The listing builds one solid part. Answer for the finished solid, in the listing's coordinates (mm). A direction names the side the tool comes from. Give positions to 0.01 mm unless a question says otherwise; leave off trailing zeros. Write each loop counter-clockwise with the first axis right and the second up, starting at its lowest first coordinate (ties: lowest second). Pieces come first, ordered by that corner, then holes. Notation, with made-up numbers: M -38.5,26.25 L -13.5,26.25 A26 ccw -13.5,43.25 Z; hole C 73.25,26.5 d9. An arc over 180 degrees is marked long. Answer as a JSON object with one key per item and string values.
```python
from build123d import *

# Parameters (mm, degrees)
BOSS_EXTRUDE1_DEPTH     = 50
BOSS_EXTRUDE1_2_DEPTH   = 50
BOSS_EXTRUDE2_DEPTH     = 10
CHAMFER1_SIZE           = 15
CHAMFER1_SIZE_2         = 20
SKETCH4_W               = 160
SKETCH4_H               = 200
BOSS_EXTRUDE3_DEPTH     = 5
FILLET1_R               = 10
SKETCH5_R               = 7.5
CUT_EXTRUDE1_DEPTH      = 5
CUT_EXTRUDE5_DEPTH      = 140.373598648
CUT_EXTRUDE5_DEPTH_BACK = 140.373598648
FILLET4_R               = 5
SKETCH12_R              = 2
CUT_EXTRUDE6_DEPTH      = 10


with BuildPart() as part:
    # Sketch2 → Boss-Extrude1 (new body)
    with BuildSketch(Plane.XY):
        with BuildLine():
            Line((-50, 75), (-22.70223243, 0))
            Line((-22.70223243, 0), (-37.64392369, -17.092022104))
            ThreePointArc((-37.64392369, -17.092022104), (-49.971924127, -51.675350432), (-35.355339059, -85.355339059))
            Line((-35.355339059, -85.355339059), (-35.355339059, -100))
            Line((-35.355339059, -100), (-80, -100))
            Line((-80, -100), (-80, 100))
            Line((-80, 100), (-50, 100))
            Line((-50, 100), (-50, 75))
        make_face()
    extrude(amount=-BOSS_EXTRUDE1_DEPTH)



with BuildPart() as body_2:
    # Sketch2 → Boss-Extrude1 2 (new body)
    with BuildSketch(Plane.XY):
        with BuildLine():
            Line((50, 75), (22.70223243, 0))
            Line((22.70223243, 0), (37.64392369, -17.092022104))
            ThreePointArc((37.64392369, -17.092022104), (49.971924127, -51.675350432), (35.355339059, -85.355339059))
            Line((35.355339059, -85.355339059), (35.355339059, -100))
            Line((35.355339059, -100), (80, -100))
            Line((80, -100), (80, 100))
            Line((80, 100), (50, 100))
            Line((50, 100), (50, 75))
        make_face()
    extrude(amount=-BOSS_EXTRUDE1_2_DEPTH)


with BuildPart() as part_1:
    add(part.part)

    add(body_2.part)  # Boss-Extrude2 merges body 2
    # Sketch3 → Boss-Extrude2 (add)
    with BuildSketch(Plane.XY):
        Polygon((-29.981637115, 20), (29.981637115, 20), (22.70223243, 0), (-22.70223243, 0), align=None)
    extrude(amount=-BOSS_EXTRUDE2_DEPTH)

    # Chamfer1
    # the kernel refuses this chamfer: 20, 15 mm, written as the material it takes off along each edge
    with BuildSketch(Plane(origin=(-81.595588718, 20, -10), x_dir=(0, 0.041308380137954244, 0.9991464445867674), z_dir=(1, 0, 0))) as chamfer1_piece_1_section:
        Polygon((CHAMFER1_SIZE * 0.999146444587, CHAMFER1_SIZE * 0.041308380138), (-CHAMFER1_SIZE_2 * 0.041308380138, CHAMFER1_SIZE_2 * 0.999146444587), (0, 0), align=None)
    chamfer1_piece_1 = extrude(amount=163.191177435, mode=Mode.PRIVATE)
    chamfer1_piece_1 = split(chamfer1_piece_1, bisect_by=Plane(origin=(-24.447399798, 4.794807938, -4.975922198), z_dir=(0.9396926207859094, 0.3420201433256661, 0)), keep=Keep.TOP, mode=Mode.PRIVATE)
    chamfer1_piece_1 = split(chamfer1_piece_1, bisect_by=Plane(origin=(24.447399798, 4.794807938, -4.975922198), z_dir=(-0.939692620785907, 0.34202014332567265, 0)), keep=Keep.TOP, mode=Mode.PRIVATE)
    add(chamfer1_piece_1, mode=Mode.SUBTRACT)

    # Sketch4 → Boss-Extrude3 (add)
    with BuildSketch(Plane.XY):
        Rectangle(SKETCH4_W, SKETCH4_H)
    extrude(amount=BOSS_EXTRUDE3_DEPTH)

    # Fillet1
    fillet1_edges = [part_1.edges().sort_by_distance(p)[0] for p in [
        (-22.70223243, 0, -30),
        (-35.355339059, -85.355339059, -25),
        (35.355339059, -85.355339059, -25),
        (22.70223243, 0, -30),
        (0, 13.333333333, 0),
    ]]
    fillet(fillet1_edges, radius=FILLET1_R)

    # Sketch5 → Cut-Extrude1 (cut)
    with BuildSketch(Plane(origin=(0, 0, 0), x_dir=(-1, 0, 0), z_dir=(0, 0, -1))):
        with Locations((0, -50)):
            Circle(SKETCH5_R)
    extrude(amount=-CUT_EXTRUDE1_DEPTH, mode=Mode.SUBTRACT)

    # Sketch11 → Cut-Extrude5 (cut, two sides: drawn at the far end of the back side and taken through both)
    with BuildSketch(Plane(origin=(0, 0, -50), x_dir=(-1, 0, 0), z_dir=(0, 0, -1)).offset(-CUT_EXTRUDE5_DEPTH_BACK)):
        with BuildLine():
            Line((-58.784198233, -62.017405631), (-51.672968794, -96.802610845))
            ThreePointArc((-51.672968794, -96.802610845), (-51.161121522, -98.466118532), (-50.338653833, -100))
            Line((-50.338653833, -100), (-80, -100))
            Line((-80, -100), (-80, 100))
            Line((-80, 100), (-62.474937186, 100))
            ThreePointArc((-62.474937186, 100), (-66.199502533, 94.806221081), (-65.536970349, 88.4494312))
            Line((-65.536970349, 88.4494312), (-60, 73.236730193))
            Line((-60, 73.236730193), (-34.120235365, 2.132661237))
            Line((-34.120235365, 2.132661237), (-45.172708428, -10.510426525))
            ThreePointArc((-45.172708428, -10.510426525), (-58.008635864, -34.670350128), (-58.784198233, -62.017405631))
        make_face()
        with BuildLine():
            Line((34.120235365, 2.132661237), (45.172708428, -10.510426525))
            ThreePointArc((45.172708428, -10.510426525), (58.008635864, -34.670350128), (58.784198233, -62.017405631))
            Line((58.784198233, -62.017405631), (51.672968794, -96.802610845))
            ThreePointArc((51.672968794, -96.802610845), (51.161121522, -98.466118532), (50.338653833, -100))
            Line((50.338653833, -100), (80, -100))
            Line((80, -100), (80, 100))
            Line((80, 100), (62.474937186, 100))
            ThreePointArc((62.474937186, 100), (66.199502533, 94.806221081), (65.536970349, 88.4494312))
            Line((65.536970349, 88.4494312), (60, 73.236730193))
            Line((60, 73.236730193), (34.120235365, 2.132661237))
        make_face()
    extrude(amount=CUT_EXTRUDE5_DEPTH + CUT_EXTRUDE5_DEPTH_BACK, mode=Mode.SUBTRACT)

    # Fillet4
    fillet4_edges = [part_1.edges().sort_by_distance(p)[0] for p in [
        (-35.355339059, -100, -25),
        (-50, 100, -25),
        (62.474937186, 100, -22.5),
        (-62.474937186, 100, -22.5),
        (50, 100, -25),
        (35.355339059, -100, -25),
    ]]
    fillet(fillet4_edges, radius=FILLET4_R)

    # Sketch12 → Cut-Extrude6 (cut)
    with BuildSketch(Plane(origin=(0, 0, -50), x_dir=(-1, 0, 0), z_dir=(0, 0, -1))):
        with Locations((-57.5, 92.5)):
            Circle(SKETCH12_R)
        with Locations((57.5, 92.5)):
            Circle(SKETCH12_R)
        with Locations((-42.855339059, -95)):
            Circle(SKETCH12_R)
        with Locations((42.855339059, -95)):
            Circle(SKETCH12_R)
    extrude(amount=-CUT_EXTRUDE6_DEPTH, mode=Mode.SUBTRACT)


solid = part_1.part
```
1. For faces 1 (the cylindrical face through (36.859, -98.574, -25.35)), 2 (the flat face through (-50, 85, -25)), 3 (the flat face through (43, -95, -40)), determine the directions among +Z, -Z, +X, -X, +Y, -Y from which every point of the face is accessible in a straight line to the end or side of a thin tool.
Verdict:
{"face 1": "-Z, -Y", "face 2": "-Z, +Y", "face 3": "-Z"}
2. A cutting plane is placed at B-B, the plane y = -50. Give the vertices of the cut face in (x, z).
Verdict:
{"outline": "M -60,-50 L -50,-50 L -50,0 L -7.5,0 L -7.5,5 L -60,5 Z; M 7.5,0 L 50,0 L 50,-50 L 60,-50 L 60,5 L 7.5,5 Z"}
3. A cutting plane is placed at D-D, the plane z = -46. Count the separate pieces of the cut face and the enclosed holes in it, plus the area to 3 significant figures.
Verdict:
{"separate pieces": "2", "enclosed holes": "4", "area": "4,740 mm2"}
4. A cutting plane is placed at C-C, the plane x = -20.5. Give the vertices of the cut face in (y, z), plus the area to 3 significant figures.
Verdict:
{"outline": "M -100,0 L 0,0 L 0,-10 L 10.67,-2 A10 cw 16.67,0 L 100,0 L 100,5 L -100,5 Z", "area": "1,070 mm2"}
5. Flat-ended cylindrical pins translate along their axes: pin 1 (6 mm diameter, centred on x = -34.5, y = 78, fed in from -Z); pin 2 (3 mm diameter, centred on y = -92, z = -14.5, fed in from -X); pin 3 (5 mm diameter, centred on x = 9.5, z = -3, fed in from -Y). Find the tip coordinate at first contact, or state that the pin passes through.
Verdict:
{"pin 1": "stops at z = 0", "pin 2": "stops at x = -52.96", "pin 3": "stops at y = 0"}
6. Consider line 1 along Y through (x, z) = (0, 2.6); line 2 along X through (y, z) = (92, -45); line 3 along X through (y, z) = (-23, -17.5). Determine where each line is inside the solid, lowest interval first.
Verdict:
{"line 1": "y = -100 to -57.5, -42.5 to 100", "line 2": "x = -66.49 to -59.44, -55.56 to -50, 50 to 55.56, 59.44 to 66.49", "line 3": "x = -53.58 to -42.08, 42.08 to 53.58"}
7. A cutting plane is placed at A-A, the plane x = 0. Give the vertices of the cut face in (y, z).
Verdict:
{"outline": "M -100,0 L -57.5,0 L -57.5,5 L -100,5 Z; M -42.5,0 L 0,0 L 0,-10 L 10.67,-2 A10 cw 16.67,0 L 100,0 L 100,5 L -42.5,5 Z"}
